```python
from build123d import *

# Parameters (mm, degrees)
F0_R     = 0.55
F1_DEPTH = 6
F2_DEPTH = 4
F3_W     = 19
F3_H     = 14
F3_W_2   = 17
F3_H_2   = 6
F4_DEPTH = 1


with BuildPart() as f1:
    # F0 (on Front) → F1 (new body)
    with BuildSketch(Plane.XZ):
        Polygon((0, 5), (0, 0), (12, 0), (12, -22), (0, -22), (0, -27), (12, -27), (17, -27), (17, 5), (12, 5), align=None)
        with Locations((6.25, -25)):
            Circle(F0_R, mode=Mode.SUBTRACT)
        with Locations((6.25, 3)):
            Circle(F0_R, mode=Mode.SUBTRACT)
    extrude(amount=F1_DEPTH)

    # F2 (add): a face of the model
    f2_faces = [f1.faces().sort_by_distance(p)[0] for p in [
        (8.5, -3, 5),
    ]]
    extrude(f2_faces, amount=F2_DEPTH)

    # F3 (on face) → F4 (join)
    with BuildSketch(Plane.XY.offset(9)):
        with Locations((8.5, -3)):
            Rectangle(F3_W, F3_H)
        with Locations((8.5, -3)):
            Rectangle(F3_W_2, F3_H_2, mode=Mode.SUBTRACT)
        with Locations((8.5, -3)):
            Rectangle(F3_W_2, F3_H_2)
    extrude(amount=F4_DEPTH)


solid = f1.part
```
Source: CAD feature listing. Evaluate the final solid. Frame: model axes, mm. A direction names the side the tool comes from. Round coordinates to 2 decimals unless told otherwise and drop trailing zeros. Loops run counter-clockwise (first coordinate to the right, second up) from the corner with the lowest first, then second, coordinate; pieces in that order, holes last. Notation, with made-up numbers: M -5.75,-36 L 23.25,-36 A21 cw 23.25,-5 Z; hole C 72.5,76.5 d2. An arc over 180 degrees is marked long. Use a Markdown table: item, result. Add a question column.
1. Set-up query: faces 5 (the flat face through (0, -3, 4)), 6 (the flat face through (12.4, 0, -9.3)), 7 (the flat face through (6, -3, -22)), 8 (the flat face through (12.4, -6, -9.3)). Return all of +Z, -Z, +X, -X, +Y, -Y with unobstructed straight access to the full face (end or side cutting, diameter ignored); none if empty.
2. Contact query for flat-ended pins moving along their axis: pin 1 (1.5 mm diameter, centred on x = 5.5, z = 6, fed in from -Y); pin 2 (3 mm diameter, centred on y = 0.5, z = -22.5, fed in from -X); pin 3 (6 mm diameter, centred on x = 12.5, z = -12, fed in from +Y). Output: stop coordinate, or through.
3. Cut plane B-B, the plane y = -5.5. Output: boundary loops of the cut face in (x, z).
4. Cut plane A-A, the plane x = 6.25. Output: boundary loops of the cut face in (y, z).
5. Ray query, line 1 along Z through (x, y) = (6.25, -1.35); line 2 along Y through (x, z) = (13, -14.5); line 3 along X through (y, z) = (-3.25, -9.5). Return the intervals inside material, ascending. Write a range as [from, to].
6. Cut plane D-D, the plane x = 10.5. Output: boundary loops of the cut face in (y, z).
7. Pull-direction query (Z, two-part tool) for faces 1 (the cylindrical face through (6.55, -2.96, -24.54)), 2 (the flat face through (8, -3, 10)), 3 (the flat face through (-1, -3.1, 9.5)), 4 (the flat face through (12, -3, -11)); classes: +Z half, -Z half, draft (parallel to the pull), parting line (faces both ways), or undercut.
8. Cut plane C-C, the plane z = 3. Output: boundary loops of the cut face in (x, y), and give its area (3 significant figures).
Solution:
| question | item | result |
|---|---|---|
| 1 | face 5 | -Z, -X, +Y, -Y |
| 1 | face 6 | -Z, +X, -X, +Y |
| 1 | face 7 | -X, +Y, -Y |
| 1 | face 8 | -Z, +X, -X, -Y |
| 2 | pin 1 | stops at y = -6 |
| 2 | pin 2 | stops at x = 0 |
| 2 | pin 3 | stops at y = 0 |
| 3 | outline | M -1,9 L 0,9 L 0,0 L 12,0 L 12,-22 L 0,-22 L 0,-27 L 17,-27 L 17,9 L 18,9 L 18,10 L -1,10 Z; hole C 6.25,-25 d1.1; hole C 6.25,3 d1.1 |
| 4 | outline | M -10,9 L -6,9 L -6,3.55 L 0,3.55 L 0,9 L 4,9 L 4,10 L -10,10 Z; M -6,-27 L 0,-27 L 0,-25.55 L -6,-25.55 Z; M -6,-24.45 L 0,-24.45 L 0,-22 L -6,-22 Z; M -6,0 L 0,0 L 0,2.45 L -6,2.45 Z |
| 5 | line 1 | z = [-27, -25.55], [-24.45, -22], [0, 2.45], [3.55, 10] |
| 5 | line 2 | y = [-6, 0] |
| 5 | line 3 | x = [12, 17] |
| 6 | outline | M -10,9 L -6,9 L -6,0 L 0,0 L 0,9 L 4,9 L 4,10 L -10,10 Z; M -6,-27 L 0,-27 L 0,-22 L -6,-22 Z |
| 7 | face 1 | undercut |
| 7 | face 2 | +Z half |
| 7 | face 3 | draft |
| 7 | face 4 | undercut |
| 8 | outline | M 0,-6 L 5.7,-6 L 5.7,0 L 0,0 Z; M 6.8,-6 L 17,-6 L 17,0 L 6.8,0 Z |
| 8 | area | 95.4 mm2 |
